Could you check a few things on this model? Use its own coordinates, in mm. Coordinates: 2 decimals unless noted, no trailing zeros. Loops run counter-clockwise (first coordinate to the right, second up) from the corner with the lowest first, then second, coordinate; pieces in that order, holes last. Notation, with made-up numbers: (26, 72.25) -> (35, 72.25) arc R21 cw to (35, 109.25) -> close; hole circle Ø8 at (15, -18.75). An arc over 180 degrees is marked (long way). One line per question, with ' | ' between items. Start each with the question number.
(1) If I drill on line 1 along Y through (x, z) = (0, 3); line 2 along Y through (x, z) = (1, 0.7), over which ranges is the centre line in solid material (lowest first)?
(2) Suppose I cut it at A-A (x = 0). Please give me the cut outline in (y, z).
(3) I'm going to push a flat-ended pin straight in: pin 1 Ø1 at (x, z) = (-2.5, 2) entering from +Y. Where does the tip first touch, or does it pass through?
(4) If we mould it in two halves opening along Y, with no side actions, what happens to faces 1 (the face through (-1.4, 0.06, 2.28)), 2 (the face through (-2.93, 2.9, 2.28)), 3 (the face through (0, -3.5, 2)), 4 (the face through (-3.5, -1, 2))? For each: pulls with the +Y half, pulls with the -Y half, needs draft (parallel to the pull), parting line crosses it, or undercut.
(5) Suppose I cut it at C-C (z = 1.6). Please give me the cut outline in (x, y).
```python
from build123d import *

# Parameters (mm, degrees)
SKETCH1_W           = 7
SKETCH1_H           = 7
BOSS_EXTRUDE1_DEPTH = 4.5
SKETCH2_R           = 1.4
CUT_EXTRUDE1_DEPTH  = 7.68954408
FILLET1_R           = 2


with BuildPart() as part:
    # Sketch1 → Boss-Extrude1 (new body)
    with BuildSketch(Plane.XY):
        Rectangle(SKETCH1_W, SKETCH1_H)
    extrude(amount=BOSS_EXTRUDE1_DEPTH)

    # Sketch2 → Cut-Extrude1 (cut, through all)
    with BuildSketch(Plane.XY.offset(4.5)):
        Circle(SKETCH2_R)
    extrude(amount=-CUT_EXTRUDE1_DEPTH, mode=Mode.SUBTRACT)

    # Fillet1
    fillet1_edges = [part.edges().sort_by_distance(p)[0] for p in [
        (-3.5, 3.5, 2.25),
    ]]
    fillet(fillet1_edges, radius=FILLET1_R)


solid = part.part
```
Checks:
1) line 1: y = -3.5 to -1.4, 1.4 to 3.5 | line 2: y = -3.5 to -0.98, 0.98 to 3.5
2) outline: (-3.5, 0) -> (-1.4, 0) -> (-1.4, 4.5) -> (-3.5, 4.5) -> close; (1.4, 0) -> (3.5, 0) -> (3.5, 4.5) -> (1.4, 4.5) -> close
3) pin 1: stops at y = 3.44
4) face 1: undercut | face 2: pulls with the +Y half | face 3: pulls with the -Y half | face 4: needs draft
5) outline: (-3.5, -3.5) -> (3.5, -3.5) -> (3.5, 3.5) -> (-1.5, 3.5) arc R2 ccw to (-3.5, 1.5) -> close; hole circle Ø2.8 at (0, 0)
